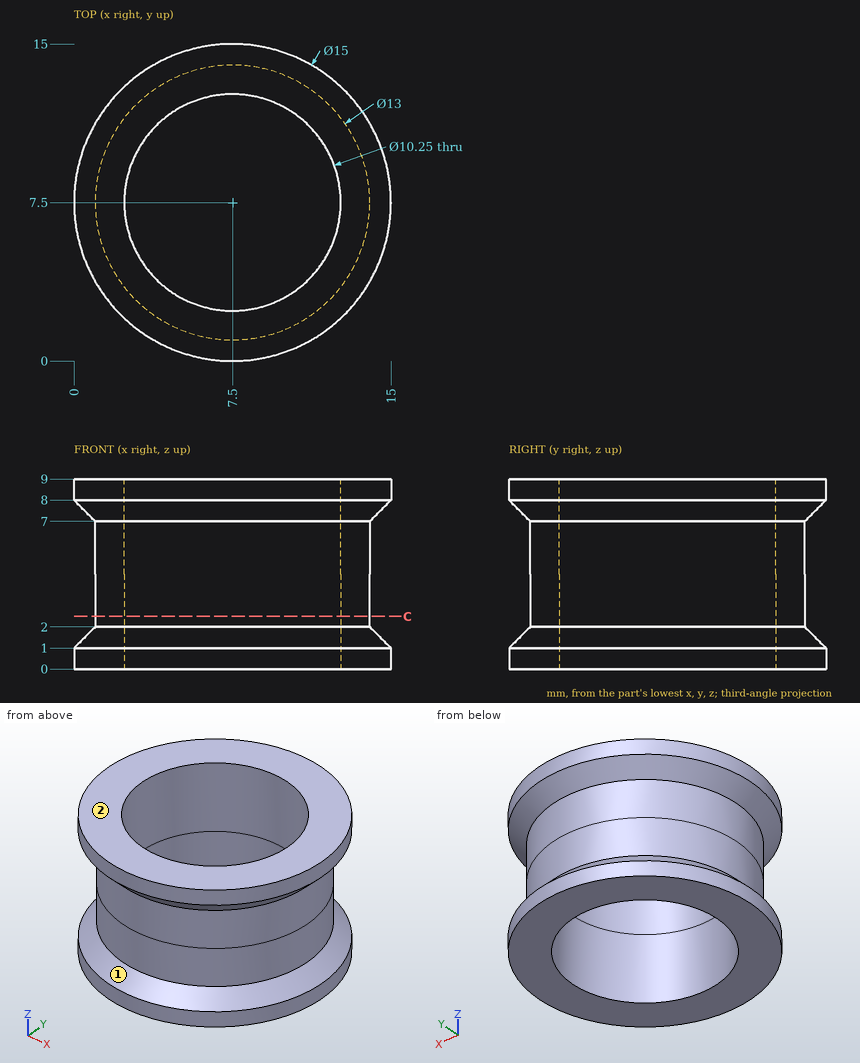
Answer from the drawing. Dimensions are ordinates in mm from the lowest x, y and z of the part. A direction names the side the tool comes from. Give positions to 0.01 mm unless a question says otherwise; leave off trailing zeros. Write each loop counter-clockwise with the first axis right and the second up, starting at its lowest first coordinate (ties: lowest second). Pieces come first, ordered by that corner, then holes.
1) A tool of negligible diameter and unlimited length cuts with its end or side. For the marked faces 1 and 2, from which of +Z, -Z, +X, -X, +Y, -Y can it reach the whole face along a straight path? Write none if from no direction.
2) Section C-C (z = 2.5) is taken. Write down the section's boundary in (x, y) (3 decimals).
3) Find the intervals of material crossed by L1, parallel to Y at x = 7.5, z = 6.45 (3 decimals); L2, parallel to Z at x = 13.5, y = 4.75; L3, parallel to X at y = 5.75, z = 1.75, in increasing order.
4) Given P1, Ø7.5, axis at x = 5.5, y = 5, coming from the -Z side; P2, Ø4, axis at x = 13.5, z = 5.5, coming from the -Y side; P3, Ø1, axis at x = 8, y = 4.5, coming from the +Z side; P4, Ø1.5, axis at y = 4, z = 7.5, coming from the -X side, each flat-ended and moving along its own axis, determine where each tip first touches the part or whether it passes through.
Response:
1. face 1: none
1. face 2: +Z, +X, -X, +Y, -Y
2. outline: circle Ø13 at (7.5, 7.5); hole circle Ø10.25 at (7.5, 7.5)
3. L1: y = 1 to 2.375, 12.625 to 14
3. L2: z = 0 to 1.9, 7.1 to 9
3. L3: x = 0.98 to 2.68, 12.32 to 14.02
4. P1: stops at z = 0
4. P2: stops at y = 2.38
4. P3: passes through
4. P4: stops at x = 0.6
